Verification items for the finished model (mm, model axes). Coordinates: 2 decimals unless noted, no trailing zeros. Write each loop counter-clockwise with the first axis right and the second up, starting at its lowest first coordinate (ties: lowest second). Pieces come first, ordered by that corner, then holes. Notation, with made-up numbers: M 62.5,-37 L 117.5,-37 A5 cw 117.5,-32 Z; hole C 25,89.5 d2. An arc over 180 degrees is marked long. Answer in a Markdown table with one row per item.
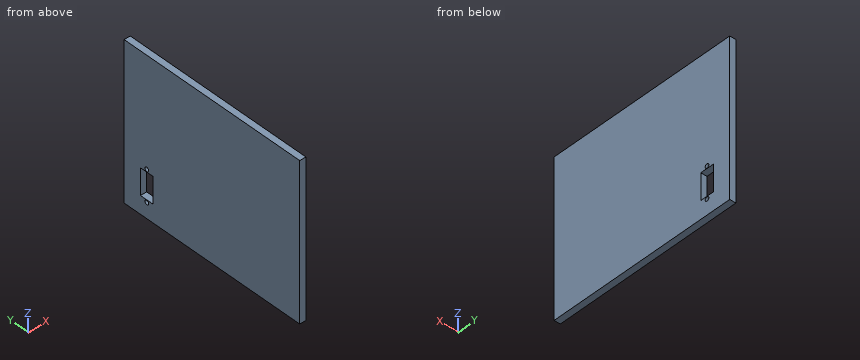
from build123d import *

# Parameters (mm, degrees)
SKETCH012_R  = 3.3
SKETCH012_W  = 22.2
SKETCH012_H  = 42.5
PAD012_DEPTH = 30
SKETCH006_W  = 310
SKETCH006_H  = 250
PAD006_DEPTH = 10


with BuildPart() as pad012:
    # Sketch012 → Pad012 (new body)
    with BuildSketch(Plane(origin=(-213, 130, 40), x_dir=(0, 1, 0), z_dir=(1, 0, 0))):
        with Locations((0, 25.3)):
            Circle(SKETCH012_R)
        with Locations((0, -25.3)):
            Circle(SKETCH012_R)
        Rectangle(SKETCH012_W, SKETCH012_H)
    extrude(amount=PAD012_DEPTH)


with BuildPart() as cut004:
    # Sketch006 → Pad006 (new body)
    with BuildSketch(Plane.YZ.offset(-210)):
        with Locations((15, 115)):
            Rectangle(SKETCH006_W, SKETCH006_H)
    extrude(amount=PAD006_DEPTH)

    # Cut004: cut Pad012
    add(pad012.part, mode=Mode.SUBTRACT)


solid = cut004.part
1) Thickness scan on L1, parallel to Z at x = -208, y = 130; L2, parallel to Y at x = -207.75, z = 14.7; L3, parallel to Y at x = -204.25, z = 41. Record the ranges inside material, lowest first. Write a range as [from, to].
Response values:
| item | result |
|---|---|
| L1 | z = [-10, 11.4], [18, 18.75], [61.25, 62], [68.6, 240] |
| L2 | y = [-140, 126.7], [133.3, 170] |
| L3 | y = [-140, 118.9], [141.1, 170] |
2) Sectioned sample at A-A (z = 35.5). Record the cut outline in (x, y).
Response values:
| item | result |
|---|---|
| outline | M -210,-140 L -200,-140 L -200,118.9 L -210,118.9 Z; M -210,141.1 L -200,141.1 L -200,170 L -210,170 Z |
3) Depth check by flat-ended pin: pin 1 (10.5 mm diameter, centred on y = 130, z = 65.3, fed in from -X); pin 2 (5.5 mm diameter, centred on y = 130, z = 14.7, fed in from +X). Enter the tip coordinate at first touch or a pass-through.
Response values:
| item | result |
|---|---|
| pin 1 | stops at x = -210 |
| pin 2 | passes through |
4) Sectioned sample at C-C (z = 65.3). Record the cut outline in (x, y).
Response values:
| item | result |
|---|---|
| outline | M -210,-140 L -200,-140 L -200,126.7 L -210,126.7 Z; M -210,133.3 L -200,133.3 L -200,170 L -210,170 Z |
5) Sectioned sample at B-B (y = 130). Record the cut outline in (x, z).
Response values:
| item | result |
|---|---|
| outline | M -210,-10 L -200,-10 L -200,11.4 L -210,11.4 Z; M -210,18 L -200,18 L -200,18.75 L -210,18.75 Z; M -210,61.25 L -200,61.25 L -200,62 L -210,62 Z; M -210,68.6 L -200,68.6 L -200,240 L -210,240 Z |
